from build123d import *

# Parameters (mm, degrees)
F4_DEPTH  = 4
F7_DEPTH  = 4
F9_R      = 5.25
F10_DEPTH = 26


with BuildPart() as f1:
    # F0 (on Front) → F1 (revolve)
    with BuildSketch(Plane.XZ):
        Polygon((-307, 17.5), (-307, 0), (307, 0), (307, 16.5), (250, 16.5), (250, 20), (195, 20), (195, 21.5), (90, 21.5), (90, 22.5), (-80, 22.5), (-80, 21.5), (-185, 21.5), (-185, 20), (-240, 20), (-240, 17.5), align=None)
    revolve(axis=Axis((0, 0, 0), (-1, 0, 0)))

    # F3 (on offset) → F4 (cut)
    with BuildSketch(Plane.XZ.offset(17.5)):
        with BuildLine():
            Line((-257, 6), (-307, 6))
            Line((-307, 6), (-307, -6))
            Line((-307, -6), (-257, -6))
            ThreePointArc((-257, -6), (-251, 0), (-257, 6))
        make_face()
    extrude(amount=-F4_DEPTH, mode=Mode.SUBTRACT)

    # F6 (on offset) → F7 (cut)
    with BuildSketch(Plane.XY.offset(16.5)):
        with BuildLine():
            Line((307, -5), (307, 5))
            Line((307, 5), (263, 5))
            ThreePointArc((263, 5), (258, 0), (263, -5))
            Line((263, -5), (307, -5))
        make_face()
    extrude(amount=-F7_DEPTH, mode=Mode.SUBTRACT)

    # F9 (on offset) → F10 (cut)
    with BuildSketch(Plane.XY.offset(22.5)):
        with Locations((-54, 0)):
            Circle(F9_R)
        with Locations((60, 0)):
            Circle(F9_R)
    extrude(amount=-F10_DEPTH, mode=Mode.SUBTRACT)


solid = f1.part
Input: part model. Units: mm. Frame: model coordinates. A direction names the side the tool comes from. Coordinates: 2 decimals unless noted, no trailing zeros. Loops run counter-clockwise (first coordinate to the right, second up) from the corner with the lowest first, then second, coordinate; pieces in that order, holes last.
Q1. Draft query along X for faces 6 (the face through (282, 0, 12.5)), 7 (the face through (60, 0, -3.5)), 8 (the face through (195, -13, -16)). Return one class per face: +X half, -X half, draft (parallel to the pull), parting line (faces both ways), or undercut.
Q2. Cut plane B-B (x = -67). Output: boundary loops of the cut face in (y, z), then the cut area to 3 significant figures.
Q3. Contact query for flat-ended pins moving along their axis: pin 1 (1 mm diameter, centred on x = 108.5, z = -8, fed in from +Y); pin 2 (3 mm diameter, centred on x = 61.5, y = -1.5, fed in from +Z); pin 3 (6 mm diameter, centred on x = -68.5, z = -15, fed in from -Y). Output: stop coordinate, or through.
Q4. Cut plane C-C (x = 60). Output: boundary loops of the cut face in (y, z).
Q5. Set-up query: faces 1 (the face through (250, 16.4, -2.9)), 2 (the face through (-133.235, 21.317, -2.799)), 3 (the face through (54.755, 0.231, 9.682)), 4 (the face through (-279, -13.5, 0)), 5 (the face through (307, 0, 0)). Return all of +Z, -Z, +X, -X, +Y, -Y with unobstructed straight access to the full face (end or side cutting, diameter ignored); none if empty.
Q6. Cut plane A-A (x = 127). Output: boundary loops of the cut face in (y, z).
Q7. Material intervals for line 1 (X direction, y = 4, z = -1.5); line 2 (X direction, y = -3, z = -16.5); line 3 (X direction, y = 18, z = -3), sorted ascending.
Working result:
1. face 6: draft
1. face 7: undercut
1. face 8: +X half
2. outline: circle Ø45 at (0, 0)
2. area: 1,590 mm2
3. pin 1: stops at y = 20.15
3. pin 2: stops at z = -3.5
3. pin 3: stops at y = -19.03
4. outline: (-5.25, -3.5) - (-5.25, 21.88) arc R22.5 ccw (long way) to (5.25, 21.88) - (5.25, -3.5) - close
5. face 1: +X
5. face 2: -X
5. face 3: +Z
5. face 4: -X, -Y
5. face 5: +Z, -Z, +X, +Y, -Y
6. outline: circle Ø43 at (0, 0)
7. line 1: x = -307 to -57.4, -50.6 to 56.6, 63.4 to 307
7. line 2: x = -307 to 250
7. line 3: x = -240 to 250
